from build123d import *

# Parameters (mm, degrees)
ENL_V_MAT_EXTRU_1_DEPTH = 7
PER_AGE2_D              = 6.8
PER_AGE2_DEPTH          = 22.25
PER_AGE2_TIP            = 2.042926105


with BuildPart() as part:
    # Esquisse1 → Base-Révolution (revolve)
    with BuildSketch(Plane.XY, mode=Mode.PRIVATE) as base_r_volution_sk:
        Polygon((-3, 0), (3, 0), (3, 7), (0, 12.196152423), (-3, 7), align=None)
    revolve(base_r_volution_sk.sketch.rotate(Axis((-10.755568754, 0, 0), (1, 0, 0)), 270), axis=Axis((-10.755568754, 0, 0), (1, 0, 0)))  # turned: the seam where the file's is

    # Esquisse2 → Enlèv. mat.-Extru.1 (cut, through all)
    with BuildSketch(Plane.ZY.offset(3)):
        Polygon((0, 19.629909152), (17, 9.814954576), (17, -9.814954576), (0, -19.629909152), (-17, -9.814954576), (-17, 9.814954576), align=None)
        Polygon((0, 8.082903769), (7, 4.041451884), (7, -4.041451884), (0, -8.082903769), (-7, -4.041451884), (-7, 4.041451884), align=None, mode=Mode.SUBTRACT)
    extrude(amount=-ENL_V_MAT_EXTRU_1_DEPTH, mode=Mode.SUBTRACT)

    # Perçage2
    with Locations(Plane(origin=(3, 0, 0), x_dir=(0, 0, -1), z_dir=(1, 0, 0))):
        with Locations((0, 0)):
            Hole(PER_AGE2_D / 2, depth=PER_AGE2_DEPTH)
            with Locations((0, 0, -(PER_AGE2_DEPTH + PER_AGE2_TIP / 2))):  # 118° drill point
                Cone(0, PER_AGE2_D / 2, PER_AGE2_TIP, mode=Mode.SUBTRACT)


solid = part.part
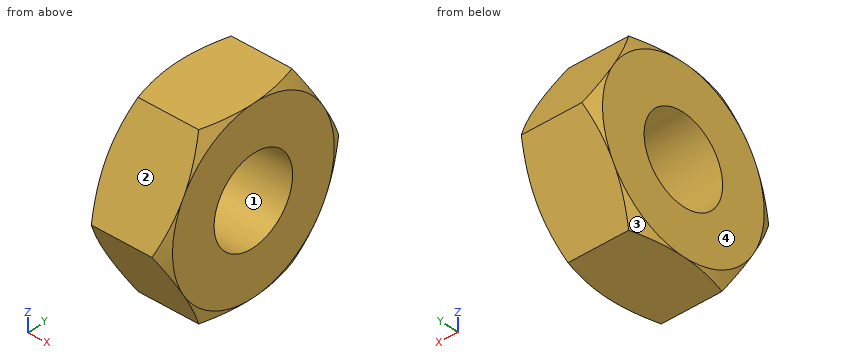
For this review, take the finished solid that the model builds, in its own axes (mm). Face numbers are marked on the shaded views. Round coordinates to 2 decimals unless told otherwise and drop trailing zeros. Write each loop counter-clockwise with the first axis right and the second up, starting at its lowest first coordinate (ties: lowest second). Pieces come first, ordered by that corner, then holes. Notation, with made-up numbers: (43.5, 49) - (53.5, 49) arc R29 cw to (53.5, 84) - close; hole circle Ø5 at (37.5, -40). An arc over 180 degrees is marked (long way). Write item = value, one per line. Start each with the question number.
1. Draft analysis for pull direction Z (two halves, no side actions). For the marked faces 1, 2, 3 and 4, state which applies: released by +Z, released by -Z, zero draft, split by the parting line, or undercut.
2. Wall thickness on L1, parallel to Z at x = 1.1, y = 1.75; L2, parallel to Z at x = -2.65, y = 2.25; L3, parallel to Y at x = 1.35, z = 2.25: over which ranges is each line inside the solid? List them lowest first.
3. Consider section A-A on x = -0.6. State the section outline as (y, z) points, plus the area to 3 significant figures.
Evaluation:
q1.face_1 = undercut
q1.face_2 = released by +Z
q1.face_3 = released by -Z
q1.face_4 = zero draft
q2.L1 = -7 to -2.92, 2.92 to 7
q2.L2 = -7 to -2.55, 2.55 to 7
q2.L3 = -6.78 to -2.55, 2.55 to 6.78
q3.outline = (-8.08, 0) - (-4.04, -7) - (4.04, -7) - (8.08, 0) - (4.04, 7) - (-4.04, 7) - close; hole circle Ø6.8 at (0, 0)
q3.area = 133 mm2
